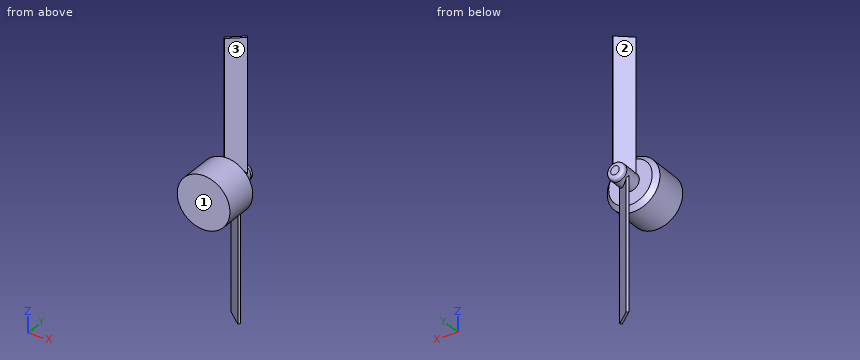
```python
from build123d import *

# Parameters (mm, degrees)
SKETCH1_R           = 11.5
BOSS_EXTRUDE1_DEPTH = 16.7
SKETCH2_R           = 2.5
BOSS_EXTRUDE2_DEPTH = 10
CHAMFER1_SIZE       = 2
SKETCH3_R           = 3.858432037
SKETCH3_R_2         = 2.5
BOSS_EXTRUDE3_DEPTH = 10
BOSS_EXTRUDE4_DEPTH = 59.69
CIRPATTERN1_COUNT   = 2
FILLET2_SIZE        = 2


with BuildPart() as part:
    # Sketch1 → Boss-Extrude1 (new body)
    with BuildSketch(Plane(origin=(0, 0, 0), x_dir=(1, 0, 0), z_dir=(0, 1, 0))):
        with Locations(Location((0, 0, 0), (0, 0, 270))):
            Circle(SKETCH1_R)
    extrude(amount=BOSS_EXTRUDE1_DEPTH)

    # Sketch2 → Boss-Extrude2 (add)
    with BuildSketch(Plane(origin=(0, 16.7, 0), x_dir=(1, 0, 0), z_dir=(0, 1, 0))):
        with Locations(Location((0, 0, 0), (0, 0, 270))):
            Circle(SKETCH2_R)
    extrude(amount=BOSS_EXTRUDE2_DEPTH)

    # Chamfer1
    chamfer1_edges = [part.edges().sort_by_distance(p)[0] for p in [
        (0, 16.7, -11.5),
    ]]
    chamfer(chamfer1_edges, length=CHAMFER1_SIZE)

    # Sketch3 → Boss-Extrude3 (add)
    with BuildSketch(Plane(origin=(0, 16.7, 0), x_dir=(1, 0, 0), z_dir=(0, 1, 0))):
        with Locations(Location((0, 0, 0), (0, 0, 270))):
            Circle(SKETCH3_R)
        Circle(SKETCH3_R_2, mode=Mode.SUBTRACT)
    extrude(amount=BOSS_EXTRUDE3_DEPTH)

    # Sketch4 → Boss-Extrude4 (add)
    with BuildSketch(Plane.XY):
        Polygon((-3.545481948, 18.385879185), (2.939679684, 23.746946134), (3.545481948, 23.014120815), (-2.939679684, 17.653053866), align=None)
    boss_extrude4 = extrude(amount=BOSS_EXTRUDE4_DEPTH)

    # CirPattern1: Boss-Extrude4 ×2 about axis
    cirpattern1_axis = Axis((0, 0, 0), (0, 1, 0))
    for i in range(1, CIRPATTERN1_COUNT):
        add(boss_extrude4.rotate(cirpattern1_axis, i * 360 / CIRPATTERN1_COUNT))

    # Fillet2
    # a fillet whose section is not a circle: 2 mm, written as the material it takes off along each edge
    with BuildSketch(Plane(origin=(0, 26.7, 0), x_dir=(0, 0, 1), z_dir=(-1, 0, 0))) as fillet2_piece_1:
        with BuildLine():
            Bezier((3.858432037, -FILLET2_SIZE), (3.858432037, 0), (3.858432037 - FILLET2_SIZE, 0), weights=[1, 1.5, 1])
            Line((3.858432037 - FILLET2_SIZE, 0), (3.858432037, 0))
            Line((3.858432037, 0), (3.858432037, -FILLET2_SIZE))
        make_face()
    revolve(axis=Axis((0, 26.7, 0), (0, 1, 0)), mode=Mode.SUBTRACT)


solid = part.part
```
Model file for the job. Use its own axes, mm. Face numbers are marked on the shaded views. Coordinates: 2 decimals unless noted, no trailing zeros. Write each loop counter-clockwise with the first axis right and the second up, starting at its lowest first coordinate (ties: lowest second). Pieces come first, ordered by that corner, then holes. Notation, with made-up numbers: (69.25, -24.5) - (94.25, -24.5) arc R4 cw to (94.25, -20.5) - close; hole circle Ø6 at (7, 14). An arc over 180 degrees is marked (long way). Use a Markdown table: item, result. Add a question column.
Item 1: Band-saw the part on A-A, the plane y = 8. Write the cut outline in (x, z), and give its area (3 significant figures).
Item 2: Band-saw the part on B-B, the plane z = -34. Write the cut outline in (x, y).
Item 3: Drill centre lines: line 1 along Z through (x, y) = (0, 25.25); line 2 along Z through (x, y) = (0.75, 14); line 3 along Y through (x, z) = (-9, 5.5). Where is each one in solid material? Low to high.
Item 4: Two-plate mould, pull along Y, no slides. Class the marked faces 1, 2 and 3: pulls with the +Y half, pulls with the -Y half, needs draft (parallel to the pull), parting line crosses it, or undercut.
Item 5: Drop flat-ended pins along their axis: pin 1 (4 mm diameter, centred on y = 9.5, z = 9.5, fed in from -X); pin 2 (10 mm diameter, centred on x = 2, y = 15, fed in from +Z); pin 3 (1.5 mm diameter, centred on y = 17, z = 45.5, fed in from -X); pin 4 (4 mm diameter, centred on y = 15.5, z = 14, fed in from +X). Give the stop position or say it passes through.
A:
| question | item | result |
|---|---|---|
| 1 | outline | circle Ø23 at (0, 0) |
| 1 | area | 415 mm² |
| 2 | outline | (-3.55, 23.01) - (2.94, 17.65) - (3.55, 18.39) - (-2.94, 23.75) - close |
| 3 | line 1 | z = -3.84 to 3.84 |
| 3 | line 2 | z = -11.48 to 11.48 |
| 3 | line 3 | y = 0 to 15.65 |
| 4 | face 1 | pulls with the -Y half |
| 4 | face 2 | pulls with the +Y half |
| 4 | face 3 | undercut |
| 5 | pin 1 | stops at x = -8.72 |
| 5 | pin 2 | stops at z = 11.5 |
| 5 | pin 3 | stops at x = -3.02 |
| 5 | pin 4 | passes through |
